```python
from build123d import *

# Parameters (mm, degrees)
F0_W     = 23.8088733172
F0_H     = 19.05
F1_DEPTH = 25.4


# Not quite as in the source:
# - ends of sketch curves that miss each other by under 0.0002 mm in the source are joined


with BuildPart() as f1:
    # F0 (on Front) → F1 (new body)
    with BuildSketch(Plane.XZ):
        Polygon((-41.275, -9.525), (41.275, -9.525), (41.275, 9.525), (22.225, 9.525), (-41.275, 9.525), align=None)
        with BuildLine():
            Line((22.225, 9.525), (41.275, 9.525))
            Line((41.275, 9.525), (41.275, 42.8498))
            Line((41.275, 42.8498), (56.2650781978, 42.8498))
            Line((56.2650781978, 42.8498), (60.325, 42.8498))
            Line((60.325, 42.8498), (60.325, 61.8998))
            Line((60.325, 61.8998), (27.8614319257, 61.8998))
            ThreePointArc((27.8614319257, 61.8998), (23.6637426323, 52.7961975559), (22.225, 42.8752))
            Line((22.225, 42.8752), (22.225, 9.525))
        make_face()
        with BuildLine():
            Line((41.275, 42.8498), (41.275, 9.525))
            add(Edge.make_bspline(
                [(56.2650781978, 42.8498), (41.47290193, 42.0072197884), (46.465802928, 20.4298387912), (41.275, 9.525)],
                knots=[0.7040277811, 0.7040277811, 0.7040277811, 0.7040277811, 36.9357748672, 36.9357748672, 36.9357748672, 36.9357748672], degree=3))
            Line((56.2650781978, 42.8498), (41.275, 42.8498))
        make_face()
        with BuildLine():
            add(Edge.make_bspline(
                [(-41.275, 9.525), (-18.2295226914, 26.9832666667), (-20.9687221795, 57.534776628), (27.8614319257, 61.8998)],
                knots=[0, 0, 0, 0, 86.7350326827, 86.7350326827, 86.7350326827, 86.7350326827], degree=3))
            Line((-41.275, 9.525), (22.225, 9.525))
            Line((22.225, 9.525), (22.225, 42.8752))
            ThreePointArc((22.225, 42.8752), (23.6637426323, 52.7961975559), (27.8614319257, 61.8998))
        make_face()
        Polygon((84.1338733172, 42.8498), (60.325, 42.8498), (60.325, 38.1), (111.125, 38.1), (111.125, 66.675), (60.325, 66.675), (60.325, 61.8998), (84.1338733172, 61.8998), align=None)
        with Locations((72.2294366586, 52.3748)):
            Rectangle(F0_W, F0_H)
    extrude(amount=F1_DEPTH)


solid = f1.part
```
Input: part model. Units: mm. Frame: model coordinates. A direction names the side the tool comes from. Coordinates: 2 decimals unless noted, no trailing zeros. Loops run counter-clockwise (first coordinate to the right, second up) from the corner with the lowest first, then second, coordinate; pieces in that order, holes last. Notation, with made-up numbers: M 80,-8 L 106,-8 A14 ccw 106,16 Z; hole C -23.5,79.25 d11. An arc over 180 degrees is marked long. One line per item, written item: value.
(1) Reachability of faces 1 (the flat face through (58, -13, 42.85)), 2 (the flat face through (-1, -13, -9.525)), 3 (the flat face through (44, -13, 61.9)), 4 (the flat face through (-41.275, -13, 0)), 5 (the flat face through (85, -13, 38.1)) from +Z, -Z, +X, -X, +Y, -Y: full face, straight path, thin tool, end or side. Return the list, or none.
Filled in:
face 1: -Z, +Y, -Y
face 2: -Z, +X, -X, +Y, -Y
face 3: +Z, -X, +Y, -Y
face 4: +Z, -Z, -X, +Y, -Y
face 5: -Z, +X, +Y, -Y
(2) Section B-B (z = 1). Output: boundary loops of the cut face in (x, y) (3 decimals), and give its area (3 significant figures).
Filled in:
outline: M -41.275,-25.4 L 41.275,-25.4 L 41.275,0 L -41.275,0 Z
area: 2,100 mm^2
(3) Pin query (flat end, axial travel): pin 1 (8 mm diameter, centred on x = 81, y = -6, fed in from -Z); pin 2 (10 mm diameter, centred on x = 2.5, y = -15, fed in from +Z); pin 3 (3 mm diameter, centred on x = 51, y = -19, fed in from -Z). Return the tip coordinate at first contact, or that it passes through.
Filled in:
pin 1: z = 38.1
pin 2: z = 57.76
pin 3: z = 40.08
(4) Section A-A (x = 76). Output: boundary loops of the cut face in (y, z) (3 decimals), and give its area (3 significant figures).
Filled in:
outline: M -25.4,38.1 L 0,38.1 L 0,66.675 L -25.4,66.675 Z
area: 726 mm^2
(5) Line query: line 1 along Z through (x, y) = (31.5, -20.75) (3 decimals); line 2 along Z through (x, y) = (93, -10.5) (3 decimals); line 3 along X through (y, z) = (-18.75, 41) (3 decimals). Output: solid intervals per line, ascending. Write a range as from..to.
Filled in:
line 1: -9.525..61.9
line 2: 38.1..66.675
line 3: -16.072..50.587, 60.325..111.125
(6) Pull-direction query (X, two-part tool) for faces 6 (the flat face through (17, -25.4, 29)), 7 (the flat face through (60.325, -13, 64)), 8 (the flat face through (60.325, -13, 41)); classes: +X half, -X half, draft (parallel to the pull), parting line (faces both ways), or undercut.
Filled in:
face 6: draft
face 7: -X half
face 8: undercut
